Check sheet for the modelled part. Datum: model origin and axes. Units: mm. Give positions to 0.01 mm unless a question says otherwise; leave off trailing zeros. Order: outer loops, then holes, each group sorted by start corner. A loop starts at its lowest first (then second) coordinate and runs counter-clockwise, first axis right, second up.
Item 1: Material ranges on line 1 along X through (y, z) = (-318, 18) (3 decimals); line 2 along Z through (x, y) = (9, -170) (3 decimals), recorded low to high.
Item 2: Sectioned sample at A-A on z = 20.25. Record the boundary of the cut face in (x, y) (3 decimals).
Item 3: Sectioned sample at C-C on x = 13. Record the boundary of the cut face in (y, z) (3 decimals), and give its area (3 significant figures).
Item 4: Sectioned sample at B-B on y = -61.5. Record the boundary of the cut face in (x, z) (3 decimals).
Item 5: Gauge pin test, flat ends, axial feed: P1, Ø16, axis at x = 21.5, y = -296.5, coming from the +Z side (3 decimals); P2, Ø4, axis at y = -321.74, z = 12.7, coming from the +X side (3 decimals). Record the tip position at first contact, or that the pin passes through.
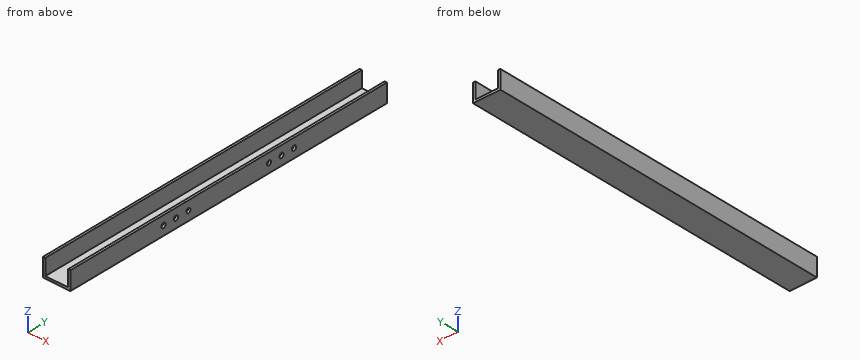
from build123d import *

# Parameters (mm, degrees)
F1_DEPTH = 482.6
F2_R     = 3.175
F3_DEPTH = 6.35


with BuildPart() as f1:
    # F0 (on Front) → F1 (new body)
    with BuildSketch(Plane.XZ):
        Polygon((0, 25.4), (0, 0), (38.1, 0), (38.1, 25.4), (34.925, 25.4), (34.925, 3.175), (3.175, 3.175), (3.175, 25.4), align=None)
    extrude(amount=F1_DEPTH)

    # F2 (on face) → F3 (cut)
    with BuildSketch(Plane.YZ.offset(38.1)):
        with Locations((-141.8082, 12.7)):
            Circle(F2_R)
        with Locations((-160.8582, 12.7)):
            Circle(F2_R)
        with Locations((-179.9082, 12.7)):
            Circle(F2_R)
        with Locations((-302.6918, 12.7)):
            Circle(F2_R)
        with Locations((-321.7418, 12.7)):
            Circle(F2_R)
        with Locations((-340.7918, 12.7)):
            Circle(F2_R)
    extrude(amount=-F3_DEPTH, mode=Mode.SUBTRACT)


solid = f1.part
Report:
1. line 1: x = 0 to 3.175, 34.925 to 38.1
1. line 2: z = 0 to 3.175
2. outline: (0, -482.6) - (3.175, -482.6) - (3.175, 0) - (0, 0) - close; (34.925, -482.6) - (38.1, -482.6) - (38.1, 0) - (34.925, 0) - close
3. outline: (-482.6, 0) - (0, 0) - (0, 3.175) - (-482.6, 3.175) - close
3. area: 1,530 mm2
4. outline: (0, 0) - (38.1, 0) - (38.1, 25.4) - (34.925, 25.4) - (34.925, 3.175) - (3.175, 3.175) - (3.175, 25.4) - (0, 25.4) - close
5. P1: stops at z = 3.175
5. P2: stops at x = 3.175
